from build123d import *

# Parameters (mm, degrees)
SKETCH1_R           = 2
SKETCH1_W           = 3.5
SKETCH1_H           = 22
SKETCH1_W_2         = 18
SKETCH1_W_3         = 20
SKETCH1_H_2         = 50
BOSS_EXTRUDE1_DEPTH = 2


with BuildPart() as part:
    # Sketch1 → Boss-Extrude1 (new body)
    with BuildSketch(Plane.XY):
        Polygon((0, -100), (-30, -96), (-35, -90), (-39, -65), (-33, -60), (-30, -54), (-30, 54), (-33, 60), (-39, 65), (-35, 90), (-30, 96), (0, 100), (30, 96), (35, 90), (39, 65), (33, 60), (30, 54), (30, -54), (33, -60), (39, -65), (35, -90), (30, -96), align=None)
        with Locations((-18, -91.5)):
            Circle(SKETCH1_R, mode=Mode.SUBTRACT)
        with Locations((-17, -81)):
            Circle(SKETCH1_R, mode=Mode.SUBTRACT)
        with Locations((-31.39400917, -82.75)):
            Circle(SKETCH1_R, mode=Mode.SUBTRACT)
        with Locations((-32.842285033, -70.837716549)):
            Circle(SKETCH1_R, mode=Mode.SUBTRACT)
        with Locations((-18.448275862, -69.087716549)):
            Circle(SKETCH1_R, mode=Mode.SUBTRACT)
        with Locations((-25, -30)):
            Circle(SKETCH1_R, mode=Mode.SUBTRACT)
        with Locations((-17.5, -18)):
            Circle(SKETCH1_R, mode=Mode.SUBTRACT)
        with Locations((0, -67)):
            Circle(SKETCH1_R, mode=Mode.SUBTRACT)
        with Locations((17.5, -18)):
            Circle(SKETCH1_R, mode=Mode.SUBTRACT)
        with Locations((25, -30)):
            Circle(SKETCH1_R, mode=Mode.SUBTRACT)
        with Locations((18.448275862, -69.087716549)):
            Circle(SKETCH1_R, mode=Mode.SUBTRACT)
        with Locations((32.842285033, -70.837716549)):
            Circle(SKETCH1_R, mode=Mode.SUBTRACT)
        with Locations((31.39400917, -82.75)):
            Circle(SKETCH1_R, mode=Mode.SUBTRACT)
        with Locations((17, -81)):
            Circle(SKETCH1_R, mode=Mode.SUBTRACT)
        with Locations((18, -91.5)):
            Circle(SKETCH1_R, mode=Mode.SUBTRACT)
        with Locations((18, 91.5)):
            Circle(SKETCH1_R, mode=Mode.SUBTRACT)
        with Locations((17, 81)):
            Circle(SKETCH1_R, mode=Mode.SUBTRACT)
        with Locations((31.39400917, 82.75)):
            Circle(SKETCH1_R, mode=Mode.SUBTRACT)
        with Locations((32.842285033, 70.837716549)):
            Circle(SKETCH1_R, mode=Mode.SUBTRACT)
        with Locations((18.448275862, 69.087716549)):
            Circle(SKETCH1_R, mode=Mode.SUBTRACT)
        with Locations((25, 30)):
            Circle(SKETCH1_R, mode=Mode.SUBTRACT)
        with Locations((17.5, 18)):
            Circle(SKETCH1_R, mode=Mode.SUBTRACT)
        with Locations((0, 67)):
            Circle(SKETCH1_R, mode=Mode.SUBTRACT)
        with Locations((-17.5, 18)):
            Circle(SKETCH1_R, mode=Mode.SUBTRACT)
        with Locations((-25, 30)):
            Circle(SKETCH1_R, mode=Mode.SUBTRACT)
        with Locations((-18.448275862, 69.087716549)):
            Circle(SKETCH1_R, mode=Mode.SUBTRACT)
        with Locations((-32.842285033, 70.837716549)):
            Circle(SKETCH1_R, mode=Mode.SUBTRACT)
        with Locations((-31.39400917, 82.75)):
            Circle(SKETCH1_R, mode=Mode.SUBTRACT)
        with Locations((-17, 81)):
            Circle(SKETCH1_R, mode=Mode.SUBTRACT)
        with Locations((-18, 91.5)):
            Circle(SKETCH1_R, mode=Mode.SUBTRACT)
        with Locations((-20.75, -49)):
            Rectangle(SKETCH1_W, SKETCH1_H, mode=Mode.SUBTRACT)
        with Locations((0, -50)):
            Rectangle(SKETCH1_W_2, SKETCH1_H, mode=Mode.SUBTRACT)
        with Locations((-20.75, 0)):
            Rectangle(SKETCH1_W, SKETCH1_H, mode=Mode.SUBTRACT)
        with Locations((20.75, 0)):
            Rectangle(SKETCH1_W, SKETCH1_H, mode=Mode.SUBTRACT)
        with Locations((20.75, -49)):
            Rectangle(SKETCH1_W, SKETCH1_H, mode=Mode.SUBTRACT)
        with Locations((20.75, 49)):
            Rectangle(SKETCH1_W, SKETCH1_H, mode=Mode.SUBTRACT)
        with Locations((0, 50)):
            Rectangle(SKETCH1_W_2, SKETCH1_H, mode=Mode.SUBTRACT)
        with Locations((-20.75, 49)):
            Rectangle(SKETCH1_W, SKETCH1_H, mode=Mode.SUBTRACT)
        Rectangle(SKETCH1_W_3, SKETCH1_H_2, mode=Mode.SUBTRACT)
    extrude(amount=BOSS_EXTRUDE1_DEPTH)


solid = part.part
The listing builds one solid part. Answer for the finished solid, in the listing's coordinates (mm). A direction names the side the tool comes from. Coordinates: 2 decimals unless noted, no trailing zeros. Order: outer loops, then holes, each group sorted by start corner. A loop starts at its lowest first (then second) coordinate and runs counter-clockwise, first axis right, second up.
Q1. Which of the six approach directions +Z, -Z, +X, -X, +Y, -Y give full straight-line access (tool end or side, diameter ignored) to faces 1 (the face through (36, 62.5, 1)), 2 (the face through (17, -79, 1)), 3 (the face through (-36, -62.5, 1))?
Q2. A cutting plane is placed at C-C, the plane z = 1.7. State how many separate pieces and enclosed holes the cut face has, and give its area (3 significant figures).
Q3. For a pull along Y with two mould halves and no side action, classify faces 4 (the face through (-15, -98, 1)), 5 (the face through (32.582, -68.855, 0.986)), 6 (the face through (15, 98, 1)) as pulls with the +Y half, pulls with the -Y half, needs draft (parallel to the pull), parting line crosses it, or undercut.
Q4. A cutting plane is placed at B-B, the plane y = 18. Write down the section's boundary in (x, z), and give its area (3 significant figures).
Q5. Consider line 1 (Y direction, x = 0, z = 1.2); line 2 (X direction, y = -10, z = 1.75); line 3 (X direction, y = -39.5, z = 1.6). Determine where each line is inside the solid, lowest interval first.
Q6. A cutting plane is placed at A-A, the plane y = -13. Write down the section's boundary in (x, z).
Q7. Given P1, Ø1, axis at x = 1, z = 1, coming from the +Y side; P2, Ø0.6, axis at y = 0.5, z = 1.5, coming from the +X side; P3, Ø1, axis at x = -15.5, z = 1, coming from the -Y side; P4, Ø2.5, axis at x = -17, y = -81, coming from the -Z side, each flat-ended and moving along its own axis, determine where each tip first touches the part or whether it passes through.
Answers follow:
1. face 1: +Z, -Z, +X
1. face 2: +Z, -Z
1. face 3: +Z, -Z, -X
2. separate pieces: 1
2. enclosed holes: 39
2. area: 10,000 mm2
3. face 4: pulls with the -Y half
3. face 5: undercut
3. face 6: pulls with the +Y half
4. outline: (-30, 0) - (-19.5, 0) - (-19.5, 2) - (-30, 2) - close; (-15.5, 0) - (-10, 0) - (-10, 2) - (-15.5, 2) - close; (10, 0) - (15.5, 0) - (15.5, 2) - (10, 2) - close; (19.5, 0) - (30, 0) - (30, 2) - (19.5, 2) - close
4. area: 64.0 mm2
5. line 1: y = -100 to -69, -65 to -61, -39 to -25, 25 to 39, 61 to 65, 69 to 100
5. line 2: x = -30 to -22.5, -19 to -10, 10 to 19, 22.5 to 30
5. line 3: x = -30 to -22.5, -19 to -9, 9 to 19, 22.5 to 30
6. outline: (-30, 0) - (-10, 0) - (-10, 2) - (-30, 2) - close; (10, 0) - (30, 0) - (30, 2) - (10, 2) - close
7. P1: stops at y = 99.93
7. P2: stops at x = 30
7. P3: stops at y = -98
7. P4: passes through
